from build123d import *

# Parameters (mm, degrees)
BOSS_EXTRUDE1_DEPTH = 200
SKETCH2_R           = 2.35
CUT_EXTRUDE1_DEPTH  = 8
CUT_EXTRUDE2_START  = -8
SKETCH3_R           = 2.35
CUT_EXTRUDE2_DEPTH  = 8
CHAMFER1_SIZE       = 1


with BuildPart() as part:
    # Sketch1 → Boss-Extrude1 (new body)
    with BuildSketch(Plane.XY):
        Polygon((-40, 40), (40, 40), (40, -40), (-40, -40), (-40, -20.45), (35, -20.45), (35, 20.45), (-40, 20.45), align=None)
    extrude(amount=BOSS_EXTRUDE1_DEPTH)

    # Sketch2 → Cut-Extrude1 (cut)
    with BuildSketch(Plane.XY.offset(200)):
        with Locations((29.5, 24.34)):
            Circle(SKETCH2_R)
        with Locations(Location((19.7, 24.34, 0), (0, 0, 180))):
            Circle(SKETCH2_R)
        with Locations((19.7, -24.34)):
            Circle(SKETCH2_R)
        with Locations(Location((29.5, -24.34, 0), (0, 0, 180))):
            Circle(SKETCH2_R)
    extrude(amount=-CUT_EXTRUDE1_DEPTH, mode=Mode.SUBTRACT)

    # Sketch3 → Cut-Extrude2 (cut)
    with BuildSketch(Plane(origin=(0, 0, 0), x_dir=(-1, 0, 0), z_dir=(0, 0, -1)).offset(CUT_EXTRUDE2_START)):
        with Locations(Location((-29.5, 24.34, 0), (0, 0, 180))):
            Circle(SKETCH3_R)
        with Locations((-19.7, 24.34)):
            Circle(SKETCH3_R)
        with Locations(Location((-19.7, -24.34, 0), (0, 0, 180))):
            Circle(SKETCH3_R)
        with Locations((-29.5, -24.34)):
            Circle(SKETCH3_R)
    extrude(amount=CUT_EXTRUDE2_DEPTH, mode=Mode.SUBTRACT)

    # Chamfer1
    chamfer1_edges = [part.edges().sort_by_distance(p)[0] for p in [
        (31.85, -24.34, 200),
        (17.35, -24.34, 200),
        (22.05, 24.34, 200),
        (27.15, 24.34, 200),
        (31.85, -24.34, 0),
        (17.35, -24.34, 0),
        (22.05, 24.34, 0),
        (27.15, 24.34, 0),
    ]]
    chamfer(chamfer1_edges, length=CHAMFER1_SIZE)


solid = part.part
Can you work these out from the model? Positions are in its coordinate system, mm. A direction names the side the tool comes from. Round coordinates to 2 decimals unless told otherwise and drop trailing zeros. Write each loop counter-clockwise with the first axis right and the second up, starting at its lowest first coordinate (ties: lowest second). Pieces come first, ordered by that corner, then holes. Notation, with made-up numbers: (-25.5, -34) - (-4.5, -34) arc R15 cw to (-4.5, -8) - close; hole circle Ø10 at (-9.75, 67.5). An arc over 180 degrees is marked (long way). Write each question's results on one line, items separated by ' | '. Start each with the question number.
1) We'd pull the mould along X, two halves only. Please class faces 1 (the flat face through (-40, -30, 99)), 2 (the cylindrical face through (30.8, 26.3, 195.5)), 3 (the flat face through (-1, 40, 99)): released by +X, released by -X, zero draft, split by the parting line, or undercut.
2) Which directions (+Z, -Z, +X, -X, +Y, -Y) give clear straight access to the entire face, cutting with the end or side of a thin tool? Please do faces 4 (the flat face through (-40, 30, 99)), 5 (the cylindrical face through (19.39, -26.67, 4.55)), 6 (the flat face through (-2, 20.45, 99)), 7 (the cylindrical face through (19.191, -26.634, 195.549)).
3) For pin 1 Ø4 at (x, y) = (19, -24) entering from +Z; pin 2 Ø10 at (x, y) = (-4.5, 18) entering from -Z; pin 3 Ø5 at (x, y) = (29, 24) entering from -Z; pin 4 Ø6 at (x, y) = (19.7, 24.34) entering from -Z, each with a flat end and sliding along its axis, tell me the tip position at first contact or that it passes through.
4) Suppose I cut it at B-B (z = 36). List the corners of the cut face in (x, y) for me.
5) Please list where these lines run through material, in increasing order: line 1 (Y direction, x = 19.7, z = 197); line 2 (X direction, y = -24, z = 195); line 3 (Y direction, x = 24.5, z = 133).
6) Suppose I cut it at C-C (x = -23). List the corners of the cut face in (y, z) for me, and give its area (3 significant figures).
7) Suppose I cut it at D-D (y = 5.5). List the corners of the cut face in (x, z) for me, and give its area (3 significant figures).
Here are the results:
1) face 1: released by -X | face 2: undercut | face 3: zero draft
2) face 4: +Z, -Z, -X, +Y, -Y | face 5: -Z | face 6: +Z, -Z, -X | face 7: +Z
3) pin 1: stops at z = 199.43 | pin 2: stops at z = 0 | pin 3: stops at z = 0.25 | pin 4: stops at z = 0.35
4) outline: (-40, -40) - (40, -40) - (40, 40) - (-40, 40) - (-40, 20.45) - (35, 20.45) - (35, -20.45) - (-40, -20.45) - close
5) line 1: y = -40 to -26.69, -21.99 to -20.45, 20.45 to 21.99, 26.69 to 40 | line 2: x = -40 to 17.37, 22.03 to 27.17, 31.83 to 40 | line 3: y = -40 to -20.45, 20.45 to 40
6) outline: (-40, 0) - (-20.45, 0) - (-20.45, 200) - (-40, 200) - close; (20.45, 0) - (40, 0) - (40, 200) - (20.45, 200) - close | area: 7,820 mm2
7) outline: (35, 0) - (40, 0) - (40, 200) - (35, 200) - close | area: 1,000 mm2
